Autodesk Inventor part; units mm, degrees
ref_plane "YZ Plane" through (0, 0, 0) normal (1, 0, 0) x (0, 1, 0)
sketch "Sketch1" plane through (0, 0, 0) normal (0, 0, 1) x (1, 0, 0)
  line L0 (-5, -9.3) -> (382, -9.3)
  line L1 (400, -27.3) -> (400, -122)
  line L2 (382, -140) -> (-400, -140)
  line L3 (-400, -140) -> (-400, -32.4)
  line L4 (-5, -9.3) -> (-5, -13.8)
  line L5 (-5, -13.8) -> (380.5, -13.8)
  line L6 (395.5, -28.8) -> (395.5, -120.5)
  line L7 (380.5, -135.5) -> (-395.5, -135.5)
  line L8 (-400, -32.4) -> (369.25, -32.4)
  line L9 (387.25, -50.4) -> (387.25, -109.25)
  line L10 (369.25, -127.25) -> (-387.25, -127.25)
  line L11 (-395.5, -135.5) -> (-395.5, -36.9)
  line L12 (-395.5, -36.9) -> (367.75, -36.9)
  line L13 (382.75, -51.9) -> (382.75, -107.75)
  line L14 (367.75, -122.75) -> (-382.75, -122.75)
  line L15 (-382.75, -122.75) -> (-382.75, -60)
  line L16 (-387.25, -127.25) -> (-387.25, -55.5)
  line L17 (-387.25, -55.5) -> (356.5, -55.5)
  line L18 (374.5, -73.5) -> (374.5, -96.5)
  line L19 (-382.75, -60) -> (355, -60)
  line L20 (370, -75) -> (370, -95)
  line L21 (355, -110) -> (-374.5, -110)
  line L22 (356.5, -114.5) -> (-374.5, -114.5)
  line L23 (-374.5, -114.5) -> (-374.5, -110)
  line L24 (323.0472, -144) -> (407.7972, -144)
  line L25 (407.7972, -144) -> (407.7972, 0)
  line L26 (407.7972, 0) -> (323.0472, 0)
  line L27 (-561.5594, 0) -> (569.3566, 0)
  line L28 (323.0472, -65) -> (345.0535, -65)
  line L29 (360.0535, -80) -> (360.0535, -90)
  line L30 (345.0535, -105) -> (323.0472, -105)
  arc A0 (360.0535, -67) -> (358.0535, -65) centre (358.0535, -67) ccw
  arc A1 (360.0535, -80) -> (345.0535, -65) centre (345.0535, -80) ccw
  arc A2 (345.0535, -105) -> (360.0535, -90) centre (345.0535, -90) ccw
  line L31 (323.0472, -18.3) -> (377.5888, -18.3)
  line L32 (377.5888, -18.3) -> (377.5888, -27.9)
  line L33 (377.5888, -27.9) -> (323.0472, -27.9)
  line L34 (323.0472, -41.4) -> (367.1423, -41.4)
  line L35 (367.1423, -41.4) -> (367.1423, -51)
  line L36 (367.1423, -51) -> (323.0472, -51)
  arc A3 (395.5, -28.8) -> (380.5, -13.8) centre (380.5, -28.8) ccw
  arc A4 (382.75, -51.9) -> (367.75, -36.9) centre (367.75, -51.9) ccw
  arc A5 (370, -75) -> (355, -60) centre (355, -75) ccw
  arc A6 (355, -110) -> (370, -95) centre (355, -95) ccw
  arc A7 (367.75, -122.75) -> (382.75, -107.75) centre (367.75, -107.75) ccw
  arc A8 (380.5, -135.5) -> (395.5, -120.5) centre (380.5, -120.5) ccw
  arc A9 (400, -27.3) -> (382, -9.3) centre (382, -27.3) ccw
  arc A10 (387.25, -50.4) -> (369.25, -32.4) centre (369.25, -50.4) ccw
  arc A11 (374.5, -73.5) -> (356.5, -55.5) centre (356.5, -73.5) ccw
  arc A12 (356.5, -114.5) -> (374.5, -96.5) centre (356.5, -96.5) ccw
  arc A13 (369.25, -127.25) -> (387.25, -109.25) centre (369.25, -109.25) ccw
  arc A14 (382, -140) -> (400, -122) centre (382, -122) ccw
  line L37 (323.0472, 0) -> (323.0472, -144)
  point P0 (0, 0)
  point P1 (400, -9.3)
  point P2 (400, -140)
  point P3 (395.5, -13.8)
  point P4 (395.5, -135.5)
  point P5 (387.25, -32.4)
  point P6 (387.25, -127.25)
  point P7 (382.75, -36.9)
  point P8 (382.75, -122.75)
  point P9 (374.5, -55.5)
  point P10 (374.5, -114.5)
  point P11 (370, -60)
  point P12 (370, -110)
  point P13 (0, 0)
  point P14 (400, -9.3)
  point P15 (400, -9.3)
  point P16 (400, -9.3)
  point P17 (395.5, -13.8)
  point P18 (395.5, -13.8)
  point P19 (395.5, -13.8)
  point P20 (387.25, -32.4)
  point P21 (387.25, -32.4)
  point P22 (387.25, -32.4)
  point P23 (382.75, -36.9)
  point P24 (382.75, -36.9)
  point P25 (382.75, -36.9)
  point P26 (374.5, -55.5)
  point P27 (374.5, -55.5)
  point P28 (374.5, -55.5)
  point P29 (370, -60)
  point P30 (370, -60)
  point P31 (370, -60)
  point P32 (370, -110)
  point P33 (370, -110)
  point P34 (370, -110)
  point P35 (374.5, -114.5)
  point P36 (374.5, -114.5)
  point P37 (374.5, -114.5)
  point P38 (382.75, -122.75)
  point P39 (382.75, -122.75)
  point P40 (382.75, -122.75)
  point P41 (387.25, -127.25)
  point P42 (387.25, -127.25)
  point P43 (387.25, -127.25)
  point P44 (395.5, -135.5)
  point P45 (395.5, -135.5)
  point P46 (395.5, -135.5)
  point P47 (400, -140)
  point P48 (400, -140)
  point P49 (400, -140)
  point P50 (360.0535, -65)
  point P51 (360.0535, -105)
  point P52 (323.0472, -13.8)
  point P53 (323.0472, -9.3)
  point P54 (323.0472, -36.9)
  point P55 (323.0472, -32.4)
  point P56 (323.0472, -140)
  point P57 (323.0472, -135.5)
  point P58 (323.0472, -110)
  point P59 (323.0472, -60)
  point P60 (323.0472, -122.75)
  point P61 (323.0472, -114.5)
  point P62 (323.0472, -55.5)
  point P63 (323.0472, -127.25)
  dimension "d91" = 0
  dimension "d1" = 4.5
  dimension "d2" = 4.5
  dimension "d3" = 4.5
  dimension "d5" = 800
  dimension "d6" = 400
  dimension "d7" = 4.5
  dimension "d8" = 4.5
  dimension "d9" = 8.25
  dimension "d10" = 4.5
  dimension "d11" = 18.6
  dimension "d12" = 4.5
  dimension "d13" = 8.25
  dimension "d14" = 4.5
  dimension "d15" = 4.5
  dimension "d16" = 4.5
  dimension "d17" = 8.25
  dimension "d19" = 18.6
  dimension "d20" = 8.25
  dimension "d88" = 4.5
  dimension "d89" = 8.25
  dimension "d90" = 8.25
  dimension "d106" = 144
  dimension "d111" = 5
  dimension "d112" = 5
  dimension "d113" = 2
  dimension "d114" = 15
  dimension "d115" = 4.5
  dimension "d116" = 4.5
  dimension "d117" = 4.5
  dimension "d118" = 4.5
  dimension "d119" = 140
  dimension "d120" = 9.3
  dimension "d121" = 15
  dimension "d122" = 18
extrude "Extrusion1" add sketch "Sketch1" along normal blind 4.5 contours L37 L26 L25 L24 L2 A14 L1 A9 L0 | L5 A3 L6 A8 L7 L37 L10 A13 L9 A10 L8 L33 L32 L31 | L12 A4 L13 A7 L14 L37 L22 A12 L18 A11 L17 L36 L35 L34 | L19 A5 L20 A6 L21 L37 L30 A2 L29 A1 L28
extrude "Extrusion7" add sketch "Sketch1" against normal blind 0.45 contours L37 L26 L25 L24 L2 A14 L1 A9 L0 | L0 A9 L1 A14 L2 L37 L7 A8 L6 A3 L5 | L5 A3 L6 A8 L7 L37 L10 A13 L9 A10 L8 L33 L32 L31 | L31 L32 L33 L37 | L8 A10 L9 A13 L10 L37 L14 A7 L13 A4 L12 | L12 A4 L13 A7 L14 L37 L22 A12 L18 A11 L17 L36 L35 L34 | L34 L35 L36 L37 | L17 A11 L18 A12 L22 L37 L21 A6 L20 A5 L19 | L19 A5 L20 A6 L21 L37 L30 A2 L29 A1 L28 | L28 A1 L29 A2 L30 L37
equation "\"d1\" = wire_diameter"
equation "\"d2\" = wire_diameter"
equation "\"d3\" = wire_diameter"
equation "\"d5\" = track_length"
equation "\"d7\" = wire_diameter"
equation "\"d8\" = wire_diameter"
equation "\"d9\" = distance_between_wires_edge"
equation "\"d10\" = wire_diameter"
equation "\"d11\" = distance_between_wires"
equation "\"d12\" = wire_diameter"
equation "\"d13\" = distance_between_wires_edge"
equation "\"d14\" = wire_diameter"
equation "\"d15\" = wire_diameter"
equation "\"d16\" = wire_diameter"
equation "\"d17\" = distance_between_wires_edge"
equation "\"d19\" = distance_between_wires"
equation "\"d20\" = distance_between_wires_edge"
equation "\"d22\" = wire_diameter"
equation "\"track_length\" = 800"
equation "\"wire_diameter\" = 4.5"
equation "\"distance_between_wires\" = -1.2 * wire_diameter + 0.2 * parameter_6"
equation "\"distance_between_wires_edge\" = 8.25"
equation "\"bend_radius\" = 15"
equation "\"bend_radius_outer\" = 18"
properties part number "primary_coil_0R2_test_cut"
Here's how the part is built. I have some questions about the finished solid (model axes, mm). A direction names the side the tool comes from. Coordinates: 2 decimals unless noted, no trailing zeros. Loops run counter-clockwise (first coordinate to the right, second up) from the corner with the lowest first, then second, coordinate; pieces in that order, holes last.
1. If we mould it in two halves opening along X, with no side actions, what happens to faces 1 (the flat face through (339, -110, 2)), 2 (the cylindrical face through (365.72, -105.49, 2.22)), 3 (the flat face through (323.047, -71, -0.2))? For each: pulls with the +X half, pulls with the -X half, needs draft (parallel to the pull), parting line crosses it, or undercut.
2. Imagine slicing it at B-B, the plane z = 1.4. Count the separate pieces of the cut face and the enclosed holes in it, and give its area (3 significant figures).
3. Imagine slicing it at A-A, the plane x = 392. Please give me the cut outline in (y, z).
4. For faces 4 (the flat face through (341, -85, 0)), 5 (the flat face through (403, -56, 4.5)), 6 (the flat face through (395.5, -74, 2)), which set-ups out of +Z, -Z, +X, -X, +Y, -Y let a thin tool reach every point of the face, with its end or its side?
5. For P1, Ø1.3, axis at y = -48, z = 3.5, coming from the -X side; P2, Ø5, axis at x = 336, y = -45, coming from the +Z side, each with a flat end and sliding along its axis, tell me the tip position at first contact or that it passes through.
6. Imagine slicing it at D-D, the plane y = -100. Please give me the cut outline in (x, z).
7. Imagine slicing it at C-C, the plane y = -15.5. Please give me the cut outline in (x, z).
8. I need wall thicknesses on L1, parallel to X at y = -89.5, z = 2.3; L2, parallel to X at y = -62, z = 3.05; L3, parallel to Y at x = 378, z = 0.4. Which ranges of each line are inside material? Lowest first, please.
Taken from the geometry:
1. face 1: needs draft
1. face 2: undercut
1. face 3: pulls with the -X half
2. separate pieces: 4
2. enclosed holes: 0
2. area: 7,110 mm2
3. outline: (-144, -0.45) - (0, -0.45) - (0, 4.5) - (-12.33, 4.5) - (-12.33, 0) - (-19.17, 0) - (-19.17, 4.5) - (-130.13, 4.5) - (-130.13, 0) - (-136.97, 0) - (-136.97, 4.5) - (-144, 4.5) - close
4. face 4: +Z, -X
4. face 5: +Z, +X, -X, +Y, -Y
4. face 6: +Z
5. P1: stops at x = 367.14
5. P2: stops at z = 0
6. outline: (323.05, -0.45) - (407.8, -0.45) - (407.8, 4.5) - (400, 4.5) - (400, 0) - (395.5, 0) - (395.5, 4.5) - (387.25, 4.5) - (387.25, 0) - (382.75, 0) - (382.75, 4.5) - (374.16, 4.5) - (374.16, 0) - (369.14, 0) - (369.14, 4.5) - (356.23, 4.5) - (356.23, 0) - (323.05, 0) - close
7. outline: (323.05, -0.45) - (407.8, -0.45) - (407.8, 4.5) - (395.59, 4.5) - (395.59, 0) - (387.44, 0) - (387.44, 4.5) - (323.05, 4.5) - close
8. L1: x = 360.05 to 370, 374.5 to 382.75, 387.25 to 395.5, 400 to 407.8
8. L2: x = 323.05 to 362.48, 370.35 to 382.75, 387.25 to 395.5, 400 to 407.8
8. L3: y = -144 to -140, -135.5 to -124.98, -118.7 to -40.95, -34.67 to -13.8, -9.3 to 0
